Here's how the part is built. I have some questions about the finished solid (model axes, mm). Round coordinates to 2 decimals unless told otherwise and drop trailing zeros. Loops run counter-clockwise (first coordinate to the right, second up) from the corner with the lowest first, then second, coordinate; pieces in that order, holes last. Notation, with made-up numbers: M -13.75,49.5 L -7.75,49.5 A20 cw -7.75,64.5 Z; hole C -32,-12.75 d1. An arc over 180 degrees is marked long. Use a Markdown table: item, result.
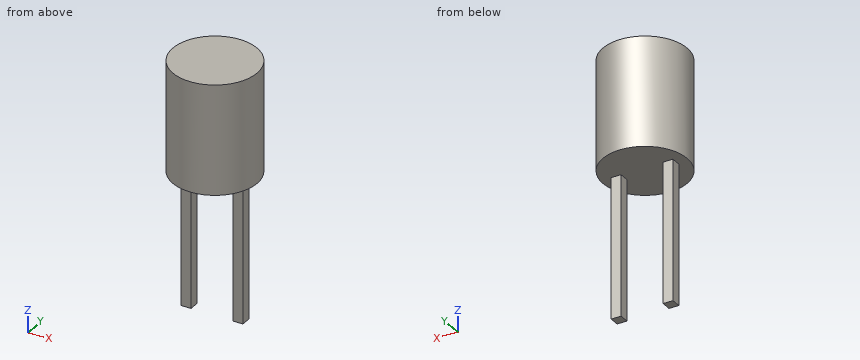
from build123d import *

# Parameters (mm, degrees)
SKETCH021_W           = 0.7
SKETCH021_H           = 0.7
PAD010002001013_DEPTH = 10
SKETCH020_R           = 3
PAD010002001012_DEPTH = 7.8


with BuildPart() as pad010002001013:
    # Sketch021 → Pad010002001013 (new body)
    with BuildSketch(Plane.XY):
        with Locations((-1.85, 0)):
            Rectangle(SKETCH021_W, SKETCH021_H)
        with Locations((1.85, 0)):
            Rectangle(SKETCH021_W, SKETCH021_H)
    extrude(amount=PAD010002001013_DEPTH)


with BuildPart() as countled:
    # Sketch020 → Pad010002001012 (new body)
    with BuildSketch(Plane.XY.offset(10)):
        Circle(SKETCH020_R)
    extrude(amount=PAD010002001012_DEPTH)

    # Fusion008: union Pad010002001013
    add(pad010002001013.part)


with BuildPart() as countled_1:
    # Fusion008 placement: moved
    add(countled.part.moved(Location((56, -5, 38))))


solid = countled_1.part
1. For pin 1 Ø0.6 at (x, z) = (58, 45.5) entering from +Y; pin 2 Ø1 at (y, z) = (-7.5, 48.5) entering from -X; pin 3 Ø0.6 at (x, z) = (58, 41) entering from -Y, each with a flat end and sliding along its axis, tell me the tip position at first contact or that it passes through.
Answer sheet:
| item | result |
|---|---|
| pin 1 | y = -4.65 |
| pin 2 | x = 53.76 |
| pin 3 | y = -5.35 |
2. Imagine slicing it at C-C, the plane x = 56. Write out the boundary of the cut face in (y, z).
Answer sheet:
| item | result |
|---|---|
| outline | M -8,48 L -2,48 L -2,55.8 L -8,55.8 Z |
3. Imagine slicing it at B-B, the plane y = -5. Write out the boundary of the cut face in (x, z), then the cut area to 3 significant figures.
Answer sheet:
| item | result |
|---|---|
| outline | M 53,48 L 53.8,48 L 53.8,38 L 54.5,38 L 54.5,48 L 57.5,48 L 57.5,38 L 58.2,38 L 58.2,48 L 59,48 L 59,55.8 L 53,55.8 Z |
| area | 60.8 mm2 |
4. I need wall thicknesses on probe 1 along X at (y, z) = (-4.7, 47); probe 2 along Z at (x, y) = (56.1, -4.2); probe 3 along Y at (x, z) = (54.2, 43). Which ranges of each line are inside material? Lowest first, please. Write a range as from..to.
Answer sheet:
| item | result |
|---|---|
| probe 1 | 53.8..54.5, 57.5..58.2 |
| probe 2 | 48..55.8 |
| probe 3 | -5.35..-4.65 |
5. Imagine slicing it at D-D, the plane z = 51.25. Write out the boundary of the cut face in (x, y), then the cut area to 3 significant figures.
Answer sheet:
| item | result |
|---|---|
| outline | C 56,-5 d6 |
| area | 28.3 mm2 |
6. Imagine slicing it at A-A, the plane z = 44. Write out the boundary of the cut face in (x, y), then the cut area to 3 significant figures.
Answer sheet:
| item | result |
|---|---|
| outline | M 53.8,-5.35 L 54.5,-5.35 L 54.5,-4.65 L 53.8,-4.65 Z; M 57.5,-5.35 L 58.2,-5.35 L 58.2,-4.65 L 57.5,-4.65 Z |
| area | 0.980 mm2 |
